Input: part model. Units: mm. Frame: model coordinates. A direction names the side the tool comes from. Coordinates: 2 decimals unless noted, no trailing zeros. Order: outer loops, then holes, each group sorted by start corner. A loop starts at its lowest first (then second) coordinate and runs counter-clockwise, first axis right, second up. Notation, with made-up numbers: (-2, 65) -> (33, 65) arc R19 cw to (33, 72) -> close; hole circle Ø11 at (13, 4). An arc over 180 degrees is marked (long way). One line per question, with ' | ' between items.
```python
from build123d import *

# Parameters (mm, degrees)
SKETCH1_W           = 25.4
SKETCH1_H           = 6.35
BOSS_EXTRUDE1_DEPTH = 12.7
SKETCH2_R           = 3.175
BOSS_EXTRUDE2_DEPTH = 3.175


with BuildPart() as part:
    # Sketch1 → Boss-Extrude1 (new body, symmetric)
    with BuildSketch(Plane.XY):
        Rectangle(SKETCH1_W, SKETCH1_H)
    extrude(amount=BOSS_EXTRUDE1_DEPTH, both=True)

    # Sketch2 → Boss-Extrude2 (add, symmetric)
    with BuildSketch(Plane.XY):
        with BuildLine():
            Line((-12.7, 3.175), (-5.493685279, 15.828674269))
            ThreePointArc((-5.493685279, 15.828674269), (0, 19.022118366), (5.493685279, 15.828674269))
            Line((5.493685279, 15.828674269), (12.7, 3.175))
            Line((12.7, 3.175), (-12.7, 3.175))
        make_face()
        with Locations((0, 12.7)):
            Circle(SKETCH2_R, mode=Mode.SUBTRACT)
    extrude(amount=BOSS_EXTRUDE2_DEPTH, both=True)


solid = part.part
```
1. Mould query, pull axis X, two halves, no side actions, for faces 4 (the face through (0, -3.175, 0)), 5 (the face through (1.5, 9.9, 0)), 6 (the face through (-12.7, 0, 0)). Classes: released by +X, released by -X, zero draft, split by the parting line, or undercut.
Recorded:
face 4: zero draft | face 5: undercut | face 6: released by -X
2. Cut plane B-B, the plane z = -1. Return loops of the section in (x, y) (3 decimals), and give its area (3 significant figures).
Recorded:
outline: (-12.7, -3.175) -> (12.7, -3.175) -> (12.7, 3.175) -> (5.494, 15.829) arc R6.322 ccw to (-5.494, 15.829) -> (-12.7, 3.175) -> close; hole circle Ø6.35 at (0, 12.7) | area: 385 mm^2
3. Access query for faces 1 (the face through (0, 3.175, -8)), 2 (the face through (0, 3.175, 8)), 3 (the face through (0, 0, 12.7)). Directions: +Z, -Z, +X, -X, +Y, -Y. A direction counts if a zero-diameter tool reaches every point of the face in a straight line with its end or side. Return the directions, or none.
Recorded:
face 1: -Z, +X, -X, +Y | face 2: +Z, +X, -X, +Y | face 3: +Z, +X, -X, +Y, -Y
4. Pin query (flat end, axial travel): pin 1 Ø1.5 at (x, z) = (-8, 0) entering from +Y; pin 2 Ø1 at (x, y) = (4, 4) entering from -Z (3 decimals); pin 3 Ø3 at (x, z) = (-2, -10) entering from +Y (3 decimals); pin 4 Ø5.5 at (x, y) = (0, 12.7) entering from +Z. Return the tip coordinate at first contact, or that it passes through.
Recorded:
pin 1: stops at y = 12.74 | pin 2: stops at z = -3.175 | pin 3: stops at y = 3.175 | pin 4: passes through
5. Cut plane C-C, the plane y = 12.7. Return loops of the section in (x, z) (3 decimals), and give its area (3 significant figures).
Recorded:
outline: (-7.275, -3.175) -> (-3.175, -3.175) -> (-3.175, 3.175) -> (-7.275, 3.175) -> close; (3.175, -3.175) -> (7.275, -3.175) -> (7.275, 3.175) -> (3.175, 3.175) -> close | area: 52.1 mm^2
6. Ray query, line 1 (Y direction, x = 0, z = 0.5) (3 decimals); line 2 (Z direction, x = -10.5, y = 5) (3 decimals). Return the intervals inside material, ascending. Write a range as [from, to].
Recorded:
line 1: y = [-3.175, 9.525], [15.875, 19.022] | line 2: z = [-3.175, 3.175]
7. Cut plane D-D, the plane z = 9.5. Return loops of the section in (x, y) (3 decimals), and give its area (3 significant figures).
Recorded:
outline: (-12.7, -3.175) -> (12.7, -3.175) -> (12.7, 3.175) -> (-12.7, 3.175) -> close | area: 161 mm^2
8. Cut plane A-A, the plane x = 0. Return loops of the section in (y, z) (3 decimals).
Recorded:
outline: (-3.175, -12.7) -> (3.175, -12.7) -> (3.175, -3.175) -> (9.525, -3.175) -> (9.525, 3.175) -> (3.175, 3.175) -> (3.175, 12.7) -> (-3.175, 12.7) -> close; (15.875, -3.175) -> (19.022, -3.175) -> (19.022, 3.175) -> (15.875, 3.175) -> close
